Source: CAD feature listing. Evaluate the final solid. Frame: model axes, mm. A direction names the side the tool comes from. Round coordinates to 2 decimals unless told otherwise and drop trailing zeros. Answer in a Markdown table with one row per item. Add a question column.
Item 1: Set-up query: faces 1 (the face through (13, 9, 1.588)), 2 (the face through (-14, -9, 1.588)), 3 (the face through (0, 0, 0)). Return all of +Z, -Z, +X, -X, +Y, -Y with unobstructed straight access to the full face (end or side cutting, diameter ignored); none if empty.
Item 2: Contact query for flat-ended pins moving along their axis: pin 1 (3 mm diameter, centred on x = -10.5, y = 5, fed in from +Z); pin 2 (23 mm diameter, centred on x = -11, y = -11.5, fed in from +Z); pin 3 (4 mm diameter, centred on y = 2, z = 16, fed in from -X). Output: stop coordinate, or through.
Item 3: Material intervals for probe 1 along Y at (x, z) = (2, 25); probe 2 along Y at (x, z) = (-3, 25.5); probe 3 along Y at (x, z) = (19, 21.5), sorted ascending.
Item 4: Mould query, pull axis X, two halves, no side actions, for faces 4 (the face through (-5.506, -24.796, 0.783)), 5 (the face through (4.587, -9.533, 14.117)), 6 (the face through (-4.587, 9.533, 14.117)), 7 (the face through (0, 0, 33.338)). Classes: released by +X, released by -X, zero draft, split by the parting line, or undercut.
from build123d import *

# Parameters (mm, degrees)
F0_R            = 25.4
F1_DEPTH        = 1.5875
F2_R            = 1.5875
F3_DEPTH        = 31.75
F5_DEPTH        = 0.79375
F5_COPIES_COUNT = 6


# Not quite as in the source:
# - a pattern or mirror of a feature is missing from the dataset's text; its kind, count and spacing are read off the source's solid


with BuildPart() as f1:
    # F0 (on Top) → F1 (new body)
    with BuildSketch(Plane.XY):
        Circle(F0_R)
    extrude(amount=F1_DEPTH)

    # F2 (on face) → F3 (join)
    with BuildSketch(Plane.XY.offset(1.5875)):
        Circle(F2_R)
    extrude(amount=F3_DEPTH)

    # F4 (on Front) → F5 (join, symmetric)
    with BuildSketch(Plane.XZ):
        with BuildLine():
            Line((1.016, 33.3375), (1.016, 1.5875))
            Line((1.016, 1.5875), (25.4, 1.5875))
            add(Edge.make_bspline(
                [(1.016, 33.3375), (22.407008335, 27.4323299527), (23.2129693031, 15.8802140504), (25.4, 1.5875)],
                knots=[0, 0, 0, 0, 40.0330108286, 40.0330108286, 40.0330108286, 40.0330108286], degree=3))
        make_face()
    f5 = extrude(amount=F5_DEPTH, both=True)

    # F5_copies: F5 ×6 about axis
    f5_copies_axis = Axis((0, 0, 0), (0, 0, 1))
    for i in range(1, F5_COPIES_COUNT):
        add(f5.rotate(f5_copies_axis, i * 360 / F5_COPIES_COUNT))


solid = f1.part
Results below:
| question | item | result |
|---|---|---|
| 1 | face 1 | +Z, +X |
| 1 | face 2 | +Z, -X |
| 1 | face 3 | -Z, +X, -X, +Y, -Y |
| 2 | pin 1 | z = 1.59 |
| 2 | pin 2 | z = 32.32 |
| 2 | pin 3 | x = -23 |
| 3 | probe 1 | -5.05 to -1.88, -0.79 to 0.79, 1.88 to 5.05 |
| 3 | probe 2 | -6.78 to -3.61, -0.79 to 0.79, 3.61 to 6.78 |
| 3 | probe 3 | -0.79 to 0.79 |
| 4 | face 4 | split by the parting line |
| 4 | face 5 | undercut |
| 4 | face 6 | undercut |
| 4 | face 7 | zero draft |
